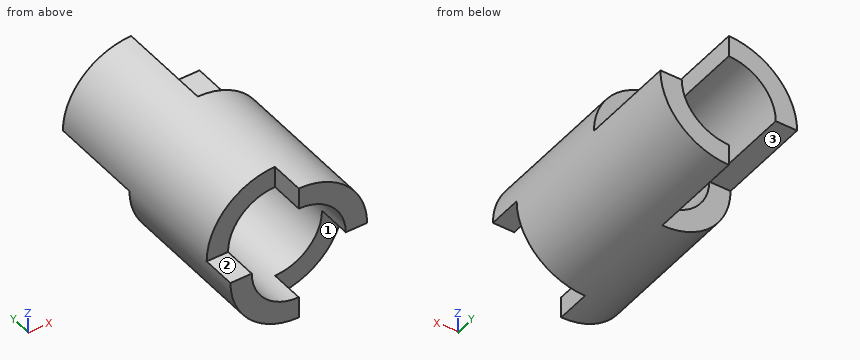
from build123d import *

# Parameters (mm, degrees)
SCHIZZO1_R                   = 4
SCHIZZO1_R_2                 = 2.75
ESTRUSIONE_ESTRUSIONE2_DEPTH = 14.1
TAGLIO_ESTRUSIONE1_DEPTH     = 5.6
TAGLIO_ESTRUSIONE2_DEPTH     = 2


with BuildPart() as part:
    # Schizzo1 → Estrusione-Estrusione2 (new body)
    with BuildSketch(Plane(origin=(0, 0, 0), x_dir=(1, 0, 0), z_dir=(0, 1, 0))):
        Circle(SCHIZZO1_R)
        Circle(SCHIZZO1_R_2, mode=Mode.SUBTRACT)
    extrude(amount=ESTRUSIONE_ESTRUSIONE2_DEPTH)

    # Schizzo2 → Taglio-Estrusione1 (cut)
    with BuildSketch(Plane(origin=(0, 14.1, 0), x_dir=(1, 0, 0), z_dir=(0, 1, 0))):
        with BuildLine():
            Line((0, 2.75), (0, 4))
            ThreePointArc((0, 4), (-2.828427125, 2.828427125), (-4, 0))
            Line((-4, 0), (-2.75, 0))
            ThreePointArc((-2.75, 0), (-1.944543648, 1.944543648), (0, 2.75))
        make_face()
        with BuildLine():
            Line((2.75, 0), (4, 0))
            ThreePointArc((4, 0), (2.828427125, -2.828427125), (0, -4))
            Line((0, -4), (0, -2.75))
            ThreePointArc((0, -2.75), (1.944543648, -1.944543648), (2.75, 0))
        make_face()
    extrude(amount=-TAGLIO_ESTRUSIONE1_DEPTH, mode=Mode.SUBTRACT)

    # Schizzo3 → Taglio-Estrusione2 (cut)
    with BuildSketch(Plane.XZ):
        with BuildLine():
            Line((0, 2.75), (0, 4))
            ThreePointArc((0, 4), (-2.828427125, 2.828427125), (-4, 0))
            Line((-4, 0), (-2.75, 0))
            ThreePointArc((-2.75, 0), (-1.944543648, 1.944543648), (0, 2.75))
        make_face()
        with BuildLine():
            Line((2.75, 0), (4, 0))
            ThreePointArc((4, 0), (2.828427125, -2.828427125), (0, -4))
            Line((0, -4), (0, -2.75))
            ThreePointArc((0, -2.75), (1.944543648, -1.944543648), (2.75, 0))
        make_face()
    extrude(amount=-TAGLIO_ESTRUSIONE2_DEPTH, mode=Mode.SUBTRACT)


solid = part.part
Verification items for the finished model (mm, model axes). Face numbers are marked on the shaded views. A direction names the side the tool comes from. Round coordinates to 2 decimals unless told otherwise and drop trailing zeros. Write each loop counter-clockwise with the first axis right and the second up, starting at its lowest first coordinate (ties: lowest second). Pieces come first, ordered by that corner, then holes.
(1) Depth check by flat-ended pin: pin 1 Ø2 at (x, z) = (1.5, 1.5) entering from +Y; pin 2 Ø1.5 at (x, z) = (2, -1.5) entering from -Y; pin 3 Ø1.5 at (y, z) = (4, -1) entering from +X; pin 4 Ø4.5 at (x, z) = (0, 0) entering from -Y. Enter the tip coordinate at first touch or a pass-through.
Returned:
pin 1: stops at y = 8.5
pin 2: stops at y = 2
pin 3: stops at x = 3.99
pin 4: passes through
(2) Access from +Z, -Z, +X, -X, +Y, -Y to the whole of each face (thin tool, end or side, straight path). Record for the marked faces 1, 2 and 3.
Returned:
face 1: -Z, +X, -Y
face 2: +Z, -X, -Y
face 3: -Z, -X, +Y
(3) Material ranges on line 1 (X direction, y = 6.5, z = 0); line 2 (X direction, y = 4.75, z = 1), recorded low to high.
Returned:
line 1: x = -4 to -2.75, 2.75 to 4
line 2: x = -3.87 to -2.56, 2.56 to 3.87
(4) Section check C-C (z = 3.25). Enter the section's corners in (x, y), plus the area to 3 significant figures.
Returned:
outline: (-2.33, 2) - (0, 2) - (0, 0) - (2.33, 0) - (2.33, 8.5) - (0, 8.5) - (0, 14.1) - (-2.33, 14.1) - close
area: 48.0 mm2
(5) Section check B-B (x = -2). Enter the section's corners in (y, z), plus the area to 3 significant figures.
Returned:
outline: (0, -3.46) - (8.5, -3.46) - (8.5, -1.89) - (0, -1.89) - close; (2, 1.89) - (14.1, 1.89) - (14.1, 3.46) - (2, 3.46) - close
area: 32.5 mm2
(6) Section check A-A (y = 11). Enter the section's corners in (x, z), plus the area to 3 significant figures.
Returned:
outline: (-4, 0) - (-2.75, 0) arc R2.75 cw to (0, 2.75) - (0, 4) arc R4 ccw to start; (0, -4) arc R4 ccw to (4, 0) - (2.75, 0) arc R2.75 cw to (0, -2.75) - close
area: 13.3 mm2
(7) Section check D-D (y = 3). Enter the section's corners in (x, z), plus the area to 3 significant figures.
Returned:
outline: circle Ø8 at (0, 0); hole circle Ø5.5 at (0, 0)
area: 26.5 mm2
